Geometry: see drawing. Coordinates: mm, zero at the bounding-box minimum. Coordinates: 2 decimals unless noted, no trailing zeros. Loops run counter-clockwise (first coordinate to the right, second up) from the corner with the lowest first, then second, coordinate; pieces in that order, holes last. Notation, with made-up numbers: (-24.5, 17.5) - (27.5, 17.5) arc R11 ccw to (27.5, 32.5) - close; hole circle Ø7 at (-16.75, -8.5). An arc over 180 degrees is marked (long way). Answer in a Markdown table with one row per item.
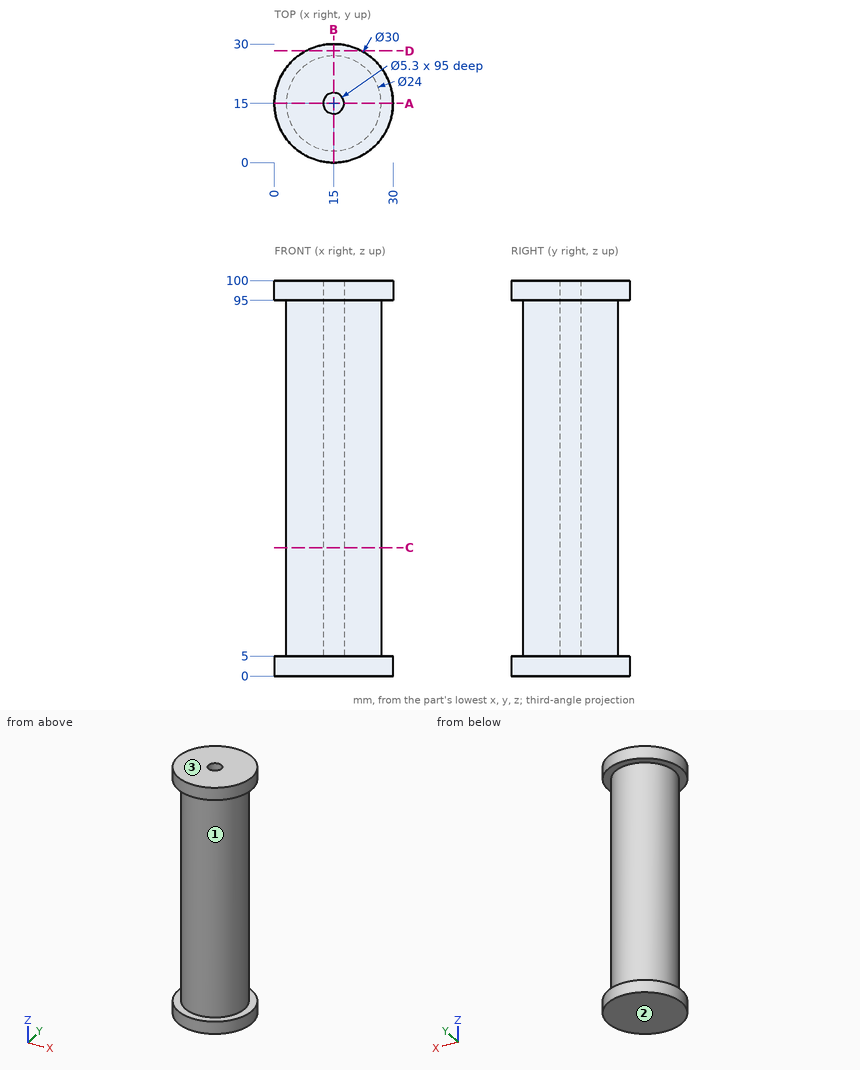
(1) First-contact query: pin 1 Ø2 at (y, z) = (10.5, 44) entering from +X; pin 2 Ø12 at (x, z) = (6, 21) entering from +Y; pin 3 Ø2 at (x, z) = (23.5, 82) entering from -Y. Flat tips, straight axial feed; report the tip coordinate or a pass-through.
Verdict:
| item | result |
|---|---|
| pin 1 | stops at x = 26.48 |
| pin 2 | stops at y = 26.62 |
| pin 3 | stops at y = 5.63 |
(2) Cut plane C-C on z = 32.5. Output: boundary loops of the cut face in (x, y).
Verdict:
| item | result |
|---|---|
| outline | circle Ø24 at (15, 15); hole circle Ø5.3 at (15, 15) |
(3) Cut plane A-A on y = 15. Output: boundary loops of the cut face in (x, z), then the cut area to 3 significant figures.
Verdict:
| item | result |
|---|---|
| outline | (0, 0) - (30, 0) - (30, 5) - (27, 5) - (27, 95) - (30, 95) - (30, 100) - (17.65, 100) - (17.65, 5) - (12.35, 5) - (12.35, 100) - (0, 100) - (0, 95) - (3, 95) - (3, 5) - (0, 5) - close |
| area | 1,960 mm² |
(4) Cut plane D-D on y = 28.25. Output: boundary loops of the cut face in (x, z).
Verdict:
| item | result |
|---|---|
| outline | (7.97, 0) - (22.03, 0) - (22.03, 5) - (7.97, 5) - close; (7.97, 95) - (22.03, 95) - (22.03, 100) - (7.97, 100) - close |
(5) Pull-direction query (Z, two-part tool) for the marked faces 1, 2 and 3; classes: pulls with the +Z half, pulls with the -Z half, needs draft (parallel to the pull), parting line crosses it, or undercut.
Verdict:
| item | result |
|---|---|
| face 1 | undercut |
| face 2 | pulls with the -Z half |
| face 3 | pulls with the +Z half |
(6) Ray query, probe 1 along Y at (x, z) = (15, 48); probe 2 along Z at (x, y) = (29.25, 18.25). Return the intervals inside material, ascending.
Verdict:
| item | result |
|---|---|
| probe 1 | y = 3 to 12.35, 17.65 to 27 |
| probe 2 | z = 0 to 5, 95 to 100 |
